from build123d import *

# Parameters (mm, degrees)
CROQUIS1_W                = 20
CROQUIS1_H                = 20
CROQUIS1_R                = 4
SALIENTE_EXTRUIR1_DEPTH   = 3
TALADRO_ROSCADO_M3X0_52_D = 2.5
REDONDEO1_R               = 5


with BuildPart() as part:
    # Croquis1 → Saliente-Extruir1 (new, symmetric)
    with BuildSketch(Plane(origin=(0, 0, 0), x_dir=(1, 0, 0), z_dir=(0, 1, 0))):
        Rectangle(CROQUIS1_W, CROQUIS1_H)
        with Locations(Location((0, 0, 0), (0, 0, 270))):
            Circle(CROQUIS1_R, mode=Mode.SUBTRACT)
    extrude(amount=SALIENTE_EXTRUIR1_DEPTH, both=True)

    # Taladro roscado M3x0.52 (through all)
    with Locations(Plane(origin=(0, 3, 0), x_dir=(1, 0, 0), z_dir=(0, 1, 0))):
        with Locations((6, 6), (-6, 6), (-6, -6), (6, -6)):
            Hole(TALADRO_ROSCADO_M3X0_52_D / 2)

    # Redondeo1
    redondeo1_edges = [part.edges().sort_by_distance(p)[0] for p in [
        (10, 0, 10),
        (-10, 0, 10),
        (-10, 0, -10),
        (10, 0, -10),
    ]]
    fillet(redondeo1_edges, radius=REDONDEO1_R)


solid = part.part
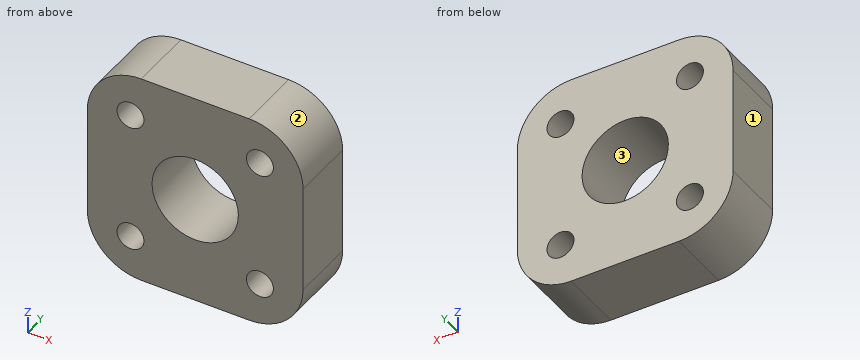
Input: part model. Units: mm. Frame: model coordinates. Face numbers are marked on the shaded views. Coordinates: 2 decimals unless noted, no trailing zeros. Order: outer loops, then holes, each group sorted by start corner. A loop starts at its lowest first (then second) coordinate and runs counter-clockwise, first axis right, second up. Notation, with made-up numbers: M 69.25,72.25 L 125.25,72.25 A30 ccw 125.25,111.25 Z; hole C 45.25,17.25 d10. An arc over 180 degrees is marked long. Answer in a Markdown table with one row per item.
(1) Section query D-D, the plane x = 6. Output: boundary loops of the cut face in (y, z), plus the area to 3 significant figures.
Numbers:
| item | result |
|---|---|
| outline | M -3,-9.9 L 3,-9.9 L 3,-7.25 L -3,-7.25 Z; M -3,-4.75 L 3,-4.75 L 3,4.75 L -3,4.75 Z; M -3,7.25 L 3,7.25 L 3,9.9 L -3,9.9 Z |
| area | 88.8 mm^2 |
(2) Contact query for a flat-ended pin moving along its axis: pin 1 Ø7 at (x, z) = (0, 0) entering from -Y. Output: stop coordinate, or through.
Numbers:
| item | result |
|---|---|
| pin 1 | passes through |
(3) Material intervals for line 1 (X direction, y = 0.9, z = -6); line 2 (X direction, y = -0.2, z = -6.25), sorted ascending. Write a range as [from, to].
Numbers:
| item | result |
|---|---|
| line 1 | x = [-9.9, -7.25], [-4.75, 4.75], [7.25, 9.9] |
| line 2 | x = [-9.84, -7.22], [-4.78, 4.78], [7.22, 9.84] |
(4) Draft query along X for the marked faces 1, 2 and 3. Return one class per face: pulls with the +X half, pulls with the -X half, needs draft (parallel to the pull), parting line crosses it, or undercut.
Numbers:
| item | result |
|---|---|
| face 1 | pulls with the -X half |
| face 2 | pulls with the +X half |
| face 3 | undercut |
(5) Section query C-C, the plane y = -0.6. Output: boundary loops of the cut face in (x, z), plus the area to 3 significant figures.
Numbers:
| item | result |
|---|---|
| outline | M -10,-5 A5 ccw -5,-10 L 5,-10 A5 ccw 10,-5 L 10,5 A5 ccw 5,10 L -5,10 A5 ccw -10,5 Z; hole C -6,-6 d2.5; hole C -6,6 d2.5; hole C 0,0 d8; hole C 6,-6 d2.5; hole C 6,6 d2.5 |
| area | 309 mm^2 |
(6) Section query A-A, the plane x = 0. Output: boundary loops of the cut face in (y, z).
Numbers:
| item | result |
|---|---|
| outline | M -3,-10 L 3,-10 L 3,-4 L -3,-4 Z; M -3,4 L 3,4 L 3,10 L -3,10 Z |
(7) Section query B-B, the plane z = 0. Output: boundary loops of the cut face in (x, y).
Numbers:
| item | result |
|---|---|
| outline | M -10,-3 L -4,-3 L -4,3 L -10,3 Z; M 4,-3 L 10,-3 L 10,3 L 4,3 Z |
